from build123d import *

# Parameters (mm, degrees)
SKETCH_1_R      = 5.276731009
SKETCH_1_R_2    = 5
EXTRUDE_1_DEPTH = 10


with BuildPart() as part:
    # 草图1 → 凸台-拉伸1 (new body)
    with BuildSketch(Plane.XY):
        Polygon((39.091663842, 5.312766173), (130.54342243, 4.388552153), (136.25140436, 9.218383017), (155.871075353, 69.515715172), (148.216212638, 77.170577887), (34.619185934, 16.543655141), align=None)
        with Locations((43.057622456, 12.073793968)):
            Circle(SKETCH_1_R, mode=Mode.SUBTRACT)
        with Locations((129.445733597, 12.073793968)):
            Circle(SKETCH_1_R, mode=Mode.SUBTRACT)
        with Locations((148.216212638, 68.164273338)):
            Circle(SKETCH_1_R_2, mode=Mode.SUBTRACT)
        Polygon((51.515213585, 15.511098763), (141.520310758, 64.87120684), (123.306992034, 15.511098763), align=None, mode=Mode.SUBTRACT)
    extrude(amount=EXTRUDE_1_DEPTH)


solid = part.part
Source: CAD feature listing. Evaluate the final solid. Frame: model axes, mm. A direction names the side the tool comes from. Coordinates: 2 decimals unless noted, no trailing zeros. Loops run counter-clockwise (first coordinate to the right, second up) from the corner with the lowest first, then second, coordinate; pieces in that order, holes last. Notation, with made-up numbers: (45, 60) - (104, 60) arc R16 cw to (104, 90) - close; hole circle Ø2 at (14, 33.5). An arc over 180 degrees is marked (long way). Return JSON: item names as keys, results as strings.
Q1. Section C-C, the plane x = 96.5. Return loops of the section in (y, z).
Results:
{"outline": "(4.73, 0) - (15.51, 0) - (15.51, 10) - (4.73, 10) - close; (40.18, 0) - (49.57, 0) - (49.57, 10) - (40.18, 10) - close"}
Q2. Contact query for flat-ended pins moving along their axis: P1, Ø8.5, axis at x = 129.45, y = 12.07, coming from the +Z side; P2, Ø5, axis at y = 65.5, z = 8.5, coming from the -X side; P3, Ø5, axis at y = 42.5, z = 1, coming from the -X side; P4, Ø5, axis at x = 86.5, z = 7.5, coming from the +Y side. Output: stop coordinate, or through.
Results:
{"P1": "through", "P2": "x = 121.66", "P3": "x = 78.57", "P4": "y = 45.57"}
Q3. Mould query, pull axis X, two halves, no side actions, for faces 3 (the cylindrical face through (47.93, 10.05, 4.93)), 4 (the flat face through (145.924, 38.945, 4.93)), 5 (the flat face through (95, 41, 0)). Classes: released by +X, released by -X, zero draft, split by the parting line, or undercut.
Results:
{"face 3": "undercut", "face 4": "released by +X", "face 5": "zero draft"}
Q4. Access query for faces 1 (the flat face through (95, 41, 10)), 2 (the flat face through (95.888, 39.846, 4.93)). Directions: +Z, -Z, +X, -X, +Y, -Y. A direction counts if a zero-diameter tool reaches every point of the face in a straight line with its end or side. Return the directions, or none.
Results:
{"face 1": "+Z, +X, -X, +Y, -Y", "face 2": "+Z, -Z"}
Q5. Section D-D, the plane z = 3. Return loops of the section in (x, y), plus the area to 3 significant figures.
Results:
{"outline": "(34.62, 16.54) - (39.09, 5.31) - (130.54, 4.39) - (136.25, 9.22) - (155.87, 69.52) - (148.22, 77.17) - close; hole circle Ø10.55 at (43.06, 12.07); hole (51.52, 15.51) - (123.31, 15.51) - (141.52, 64.87) - close; hole circle Ø10.55 at (129.45, 12.07); hole circle Ø10 at (148.22, 68.16)", "area": "2,560 mm2"}
Q6. Section A-A, the plane y = 51.5. Return loops of the section in (x, z).
Results:
{"outline": "(100.12, 0) - (117.14, 0) - (117.14, 10) - (100.12, 10) - close; (136.59, 0) - (150.01, 0) - (150.01, 10) - (136.59, 10) - close"}
Q7. Section B-B, the plane x = 128.5. Return loops of the section in (y, z), plus the area to 3 significant figures.
Results:
{"outline": "(4.41, 0) - (6.88, 0) - (6.88, 10) - (4.41, 10) - close; (17.27, 0) - (29.58, 0) - (29.58, 10) - (17.27, 10) - close; (57.73, 0) - (66.65, 0) - (66.65, 10) - (57.73, 10) - close", "area": "237 mm2"}
Q8. Material intervals for line 1 along X through (y, z) = (8.5, 4.75); line 2 along Y through (x, z) = (107.5, 0.75); line 3 along X through (y, z) = (54, 7), sorted ascending.
Results:
{"line 1": "37.82 to 39.18, 46.94 to 125.56, 133.33 to 135.4", "line 2": "4.62 to 15.51, 46.21 to 55.44", "line 3": "104.8 to 121.7, 137.51 to 150.82"}
